```python
from build123d import *

# Parameters (mm, degrees)
Y_KSEKLIK_EKSTR_ZYON2_DEPTH = 10
IZIM2_R                     = 2.5
KES_EKSTR_ZYON1_DEPTH       = 2


with BuildPart() as part:
    # Çizim1 → Yükseklik-Ekstrüzyon2 (new body)
    with BuildSketch(Plane.XY):
        with BuildLine():
            Line((-80, 0), (-80, -80))
            Line((-80, -80), (-92, -80))
            Line((-92, -80), (-92, -78))
            Line((-92, -78), (-82, -78))
            Line((-82, -78), (-82, 0))
            ThreePointArc((-82, 0), (0, 82), (82, 0))
            Line((82, 0), (82, -78))
            Line((82, -78), (92, -78))
            Line((92, -78), (92, -80))
            Line((92, -80), (80, -80))
            Line((80, -80), (80, 0))
            ThreePointArc((80, 0), (0, 80), (-80, 0))
        make_face()
    extrude(amount=Y_KSEKLIK_EKSTR_ZYON2_DEPTH)

    # Çizim2 → Kes-Ekstrüzyon1 (cut)
    with BuildSketch(Plane.XZ.offset(80)):
        with Locations(Location((87, 5, 0), (0, 0, 270))):
            Circle(IZIM2_R)
        with Locations(Location((-87, 5, 0), (0, 0, 90))):
            Circle(IZIM2_R)
    extrude(amount=-KES_EKSTR_ZYON1_DEPTH, mode=Mode.SUBTRACT)


solid = part.part
```
Source: CAD feature listing. Evaluate the final solid. Frame: model axes, mm. A direction names the side the tool comes from. Coordinates: 2 decimals unless noted, no trailing zeros. Write each loop counter-clockwise with the first axis right and the second up, starting at its lowest first coordinate (ties: lowest second). Pieces come first, ordered by that corner, then holes. Notation, with made-up numbers: (18.5, 69) -> (75.5, 69) arc R18 ccw to (75.5, 90) -> close; hole circle Ø11 at (7, -26.5). An arc over 180 degrees is marked (long way). Return JSON: item names as keys, results as strings. Group by question number.
1) Contact query for flat-ended pins moving along their axis: P1, Ø5, axis at x = 88, z = 4.5, coming from the +Y side; P2, Ø2, axis at y = 0, z = 4.5, coming from the +X side; P3, Ø6, axis at x = 26.5, z = 2.5, coming from the +Y side; P4, Ø3, axis at x = 87, z = 5, coming from the +Y side. Output: stop coordinate, or through.
2) Section query C-C, the plane y = -68. Return loops of the section in (x, z), plus the area to 3 significant figures.
3) Mould query, pull axis Z, two halves, no side actions, for faces 4 (the face through (-89.48, -79.01, 4.67)), 5 (the face through (-81, 1, 0)), 6 (the face through (-89, -78, 3)). Classes: +Z half, -Z half, draft (parallel to the pull), parting line (faces both ways), or undercut.
4) Set-up query: faces 1 (the face through (85, -78, 3)), 2 (the face through (-82, -40, 5)), 3 (the face through (-80, -39, 5)). Return all of +Z, -Z, +X, -X, +Y, -Y with unobstructed straight access to the full face (end or side cutting, diameter ignored); none if empty.
5) Section query A-A, the plane x = -87. Return loops of the section in (y, z), plus the area to 3 significant figures.
6) Section query B-B, the plane z = 5. Return loops of the section in (x, y), plus the area to 3 significant figures.
7) Section query D-D, the plane x = 0. Return loops of the section in (y, z), plus the area to 3 significant figures.
8) Ray query, line 1 along X through (y, z) = (-78.8, 5); line 2 along X through (y, z) = (-35, 6.75); line 3 along Z through (x, y) = (-87, -78.8). Return the intervals inside material, ascending.
From the geometry:
{
 "1": {"P1": "y = -78", "P2": "x = 82", "P3": "y = 78.56", "P4": "through"},
 "2": {"outline": "(-82, 0) -> (-80, 0) -> (-80, 10) -> (-82, 10) -> close; (80, 0) -> (82, 0) -> (82, 10) -> (80, 10) -> close", "area": "40.0 mm²"},
 "3": {"face 4": "undercut", "face 5": "-Z half", "face 6": "draft"},
 "4": {"face 1": "+Z, -Z, +X, +Y", "face 2": "+Z, -Z, -X, +Y", "face 3": "+Z, -Z, -Y"},
 "5": {"outline": "(-80, 0) -> (-78, 0) -> (-78, 2.5) -> (-80, 2.5) -> close; (-80, 7.5) -> (-78, 7.5) -> (-78, 10) -> (-80, 10) -> close", "area": "10.0 mm²"},
 "6": {"outline": "(-92, -80) -> (-89.5, -80) -> (-89.5, -78) -> (-92, -78) -> close; (-84.5, -80) -> (-80, -80) -> (-80, 0) arc R80 cw to (80, 0) -> (80, -80) -> (84.5, -80) -> (84.5, -78) -> (82, -78) -> (82, 0) arc R82 ccw to (-82, 0) -> (-82, -78) -> (-84.5, -78) -> close; (89.5, -80) -> (92, -80) -> (92, -78) -> (89.5, -78) -> close", "area": "849 mm²"},
 "7": {"outline": "(80, 0) -> (82, 0) -> (82, 10) -> (80, 10) -> close", "area": "20.0 mm²"},
 "8": {"line 1": "-92 to -89.5, -84.5 to -80, 80 to 84.5, 89.5 to 92", "line 2": "-82 to -80, 80 to 82", "line 3": "0 to 2.5, 7.5 to 10"}
}
